For this review, take the finished solid that the model builds, in its own axes (mm). Face numbers are marked on the shaded views. A direction names the side the tool comes from. Give positions to 0.01 mm unless a question says otherwise; leave off trailing zeros. Order: outer loops, then holes, each group sorted by start corner. A loop starts at its lowest first (then second) coordinate and runs counter-clockwise, first axis right, second up. Notation, with made-up numbers: (83.5, -35) -> (116.5, -35) arc R20 cw to (116.5, 4) -> close; hole circle Ø1 at (-34, -34). An arc over 180 degrees is marked (long way). Return JSON: item names as keys, results as strings. Group by question number.
1) The part is to be moulded in two halves that separate along Y. For the marked faces 4, 5 and 6, say which applies: released by +Y, released by -Y, zero draft, split by the parting line, or undercut.
2) Add section D-D (x = 7.5). Give the boundary of the cut face in (y, z), then the cut area to 3 significant figures.
3) Insertion check: P1, Ø1.5, axis at y = -0.5, z = -3, coming from the -X side; P2, Ø2, axis at y = -7.5, z = -0.5, coming from the +X side; P3, Ø2, axis at y = -4.5, z = -1, coming from the +X side. Each pin has a flat end and moves straight along its axis. Give the tip position at first contact, or say it passes through.
4) Add section B-B (x = 0). Give the boundary of the cut face in (y, z).
5) For the marked faces 1, 2 and 3, list the 3-axis set-ups (+Z, -Z, +X, -X, +Y, -Y) from which the entire face can be reached by the end or side of a thin tool; tool diameter is ignored.
6) Add section A-A (z = 2.25). Give the boundary of the cut face in (x, y), then the cut area to 3 significant figures.
7) To check wall thickness, follow line 1 along Y through (x, z) = (8.5, -3.5); line 2 along Y through (x, z) = (0, 0.75); line 3 along X through (y, z) = (-5.5, 3.75). State the ranges of each line that lie inside material, in increasing order.
8) Add section C-C (y = 0). Give the boundary of the cut face in (x, z).
from build123d import *

# Parameters (mm, degrees)
SKETCH_1_R      = 2.15
EXTRUDE_1_DEPTH = 4.5
FILLET_1_R      = 2
CHAMFER_1_SIZE  = 0.5
CHAMFER_1_SIZE2 = 0.508960096


with BuildPart() as part:
    # 스케치1 → 보스-돌출1 (new, symmetric)
    with BuildSketch(Plane.XY):
        with BuildLine():
            Line((-8, 0.638251315), (-5, -2.4))
            Line((-5, -2.4), (-5, -11.4))
            Line((-5, -11.4), (-2.956819065, -11.4))
            Line((-2.956819065, -11.4), (1.87605446, -6.887535593))
            Line((1.87605446, -6.887535593), (1.87605446, -4.634697365))
            ThreePointArc((1.87605446, -4.634697365), (2.999351329, -4.000486421), (3.923009049, -3.1))
            Line((3.923009049, -3.1), (9.140101739, -3.1))
            Line((9.140101739, -3.1), (14.557074242, 2.3))
            Line((14.557074242, 2.3), (14.557074242, 5.2))
            Line((14.557074242, 5.2), (11.666160546, 8.1))
            Line((11.666160546, 8.1), (6.054110701, 8.1))
            Line((6.054110701, 8.1), (6, 5))
            Line((6, 5), (-2.5, 5))
            Line((-2.5, 5), (-8, 1.878902403))
            Line((-8, 1.878902403), (-8, 0.638251315))
        make_face()
        Circle(SKETCH_1_R, mode=Mode.SUBTRACT)
    extrude(amount=EXTRUDE_1_DEPTH, both=True)

    # 필렛1
    fillet_1_edges = [part.edges().sort_by_distance(p)[0] for p in [
        (14.557074242, 2.3, 0),
    ]]
    fillet(fillet_1_edges, radius=FILLET_1_R)

    # 모따기1
    chamfer_1_edges = [part.edges().sort_by_distance(p)[0] for p in [
        (6.054110701, 8.1, 0),
    ]]
    chamfer_1_side = [part.faces().sort_by_distance(p)[0] for p in [
        (8.860135624, 8.1, 0),
    ]]
    chamfer(chamfer_1_edges, length=CHAMFER_1_SIZE, length2=CHAMFER_1_SIZE2, reference=chamfer_1_side[0])


solid = part.part
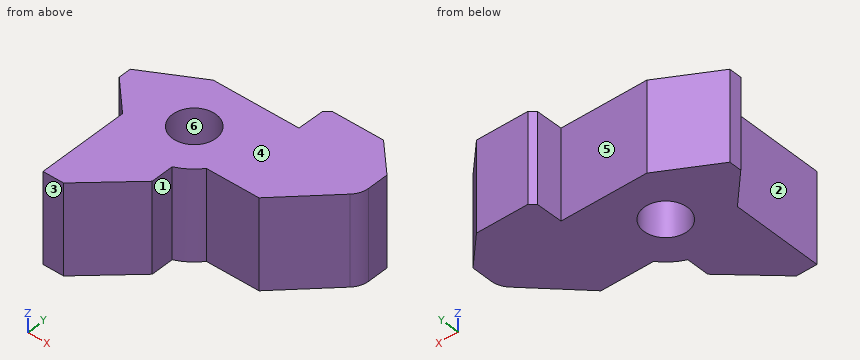
Evaluation:
{
 "1": {"face 4": "zero draft", "face 5": "released by +Y", "face 6": "undercut"},
 "2": {"outline": "(-3.1, -4.5) -> (8.1, -4.5) -> (8.1, 4.5) -> (-3.1, 4.5) -> close", "area": "101 mm^2"},
 "3": {"P1": "x = -7.62", "P2": "x = 1.88", "P3": "x = 3.57"},
 "4": {"outline": "(-8.64, -4.5) -> (-2.15, -4.5) -> (-2.15, 4.5) -> (-8.64, 4.5) -> close; (2.15, -4.5) -> (5, -4.5) -> (5, 4.5) -> (2.15, 4.5) -> close"},
 "5": {"face 1": "+Z, -Z, +X, -Y", "face 2": "+Z, -Z, -X, -Y", "face 3": "+Z, -Z, +X, -X, -Y"},
 "6": {"outline": "(-8, 0.64) -> (-5, -2.4) -> (-5, -11.4) -> (-2.96, -11.4) -> (1.88, -6.89) -> (1.88, -4.63) arc R5 ccw to (3.92, -3.1) -> (9.14, -3.1) -> (13.97, 1.71) arc R2 ccw to (14.56, 3.13) -> (14.56, 5.2) -> (11.67, 8.1) -> (6.55, 8.1) -> (6.05, 7.59) -> (6, 5) -> (-2.5, 5) -> (-8, 1.88) -> close; hole circle Ø4.3 at (0, 0)", "area": "208 mm^2"},
 "7": {"line 1": "-3.1 to 8.1", "line 2": "-8.64 to -2.15, 2.15 to 5", "line 3": "-5 to 1.88"},
 "8": {"outline": "(-7.37, -4.5) -> (-2.15, -4.5) -> (-2.15, 4.5) -> (-7.37, 4.5) -> close; (2.15, -4.5) -> (12.25, -4.5) -> (12.25, 4.5) -> (2.15, 4.5) -> close"}
}
